Verification items for the finished model (mm, model axes). Face numbers are marked on the shaded views. A direction names the side the tool comes from. Round coordinates to 2 decimals unless told otherwise and drop trailing zeros. Write each loop counter-clockwise with the first axis right and the second up, starting at its lowest first coordinate (ties: lowest second). Pieces come first, ordered by that corner, then holes.
from build123d import *

# Parameters (mm, degrees)
CHAMFER_2_SIZE = 0.1


with BuildPart() as part:
    # 草图2 → 旋转1 (revolve)
    with BuildSketch(Plane.XY, mode=Mode.PRIVATE) as revolve_1_sk:
        Polygon((3, 4), (3, 0), (6.75, 0), (6.75, 0.8), (5.8, 0.8), (5.8, 1), (6, 1), (6, 4), align=None)
    revolve(revolve_1_sk.sketch.rotate(Axis((0, 4, 0), (0, -1, 0)), 90), axis=Axis((0, 4, 0), (0, -1, 0)))

    # 倒角2
    chamfer_2_edges = [part.edges().sort_by_distance(p)[0] for p in [
        (0, 0, -6.75),
        (0, 4, -3),
        (0, 4, -6),
        (0, 1, -6),
        (0, 0.8, -6.75),
    ]]
    chamfer(chamfer_2_edges, length=CHAMFER_2_SIZE)


solid = part.part
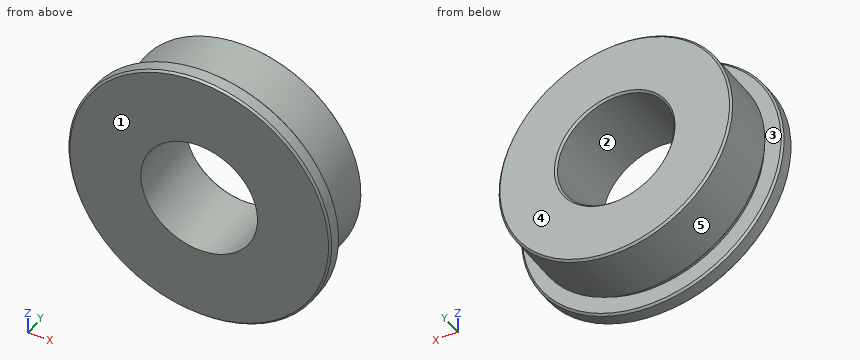
Q1. Tool access check on the marked faces 4 and 5. Record the directions out of +Z, -Z, +X, -X, +Y, -Y that give a thin tool (end or side, any length) a straight path to the whole face; none if there is none.
Recorded:
face 4: +Z, -Z, +X, -X, +Y
face 5: +Y
Q2. Depth check by flat-ended pin: P1, Ø2, axis at x = -1.5, y = 1, coming from the -Z side. Enter the tip coordinate at first touch or a pass-through.
Recorded:
P1: stops at z = -6.73
Q3. Sectioned sample at C-C (y = 2.75). Enter the section's corners in (x, z), plus the area to 3 significant figures.
Recorded:
outline: circle Ø12 at (0, 0); hole circle Ø6 at (0, 0)
area: 84.8 mm2
Q4. Sectioned sample at B-B (x = 0). Enter the section's corners in (y, z).
Recorded:
outline: (0, -6.65) - (0.1, -6.75) - (0.7, -6.75) - (0.8, -6.65) - (0.8, -5.8) - (1, -5.8) - (1, -5.9) - (1.1, -6) - (3.9, -6) - (4, -5.9) - (4, -3.1) - (3.9, -3) - (0, -3) - close; (0, 3) - (3.9, 3) - (4, 3.1) - (4, 5.9) - (3.9, 6) - (1.1, 6) - (1, 5.9) - (1, 5.8) - (0.8, 5.8) - (0.8, 6.65) - (0.7, 6.75) - (0.1, 6.75) - (0, 6.65) - close
Q5. Material ranges on line 1 along X through (y, z) = (2.85, 0); line 2 along X through (y, z) = (1.7, -2.5); line 3 along Z through (x, y) = (-1.25, 2.3), recorded low to high.
Recorded:
line 1: x = -6 to -3, 3 to 6
line 2: x = -5.45 to -1.66, 1.66 to 5.45
line 3: z = -5.87 to -2.73, 2.73 to 5.87
Q6. Release check for a two-part mould opening along Y. For the marked faces 1, 2 and 3 record: released by +Y, released by -Y, zero draft, split by the parting line, or undercut.
Recorded:
face 1: released by -Y
face 2: zero draft
face 3: undercut
Q7. Sectioned sample at A-A (z = 0). Enter the section's corners in (x, y), plus the area to 3 significant figures.
Recorded:
outline: (-6.75, 0.1) - (-6.65, 0) - (-3, 0) - (-3, 3.9) - (-3.1, 4) - (-5.9, 4) - (-6, 3.9) - (-6, 1.1) - (-5.9, 1) - (-5.8, 1) - (-5.8, 0.8) - (-6.65, 0.8) - (-6.75, 0.7) - close; (3, 0) - (6.65, 0) - (6.75, 0.1) - (6.75, 0.7) - (6.65, 0.8) - (5.8, 0.8) - (5.8, 1) - (5.9, 1) - (6, 1.1) - (6, 3.9) - (5.9, 4) - (3.1, 4) - (3, 3.9) - close
area: 25.1 mm2
